Geometry: final body of the model. Coordinates: model frame, mm. Face numbers are marked on the shaded views. Give positions to 0.01 mm unless a question says otherwise; leave off trailing zeros. Order: outer loops, then holes, each group sorted by start corner. A loop starts at its lowest first (then second) coordinate and runs counter-clockwise, first axis right, second up. Notation, with made-up numbers: (-16, -37.5) - (10, -37.5) arc R19 cw to (10, -19.5) - close; hole circle Ø3 at (66.25, -30). An arc over 180 degrees is marked (long way). One line per item, written item: value.
```python
from build123d import *

# Parameters (mm, degrees)
F1_DEPTH = 3.302
F3_DEPTH = 1.524
F4_SIZE  = 2.54
F5_DEPTH = 1.27


with BuildPart() as f1:
    # F0 (on Top) → F1 (new body)
    with BuildSketch(Plane.XY):
        Polygon((9.3258451213, 12.835924618), (-9.3258451213, 12.835924618), (-15.08953438, -4.9028869271), (0, -15.866075382), (15.08953438, -4.9028869271), align=None)
    extrude(amount=F1_DEPTH)

    # F2 (on face) → F3 (cut)
    with BuildSketch(Plane.XY.offset(3.302)):
        Polygon((7.3849782182, 10.1645505026), (-7.3849782182, 10.1645505026), (-11.9491457632, -3.8825128116), (0, -12.564075382), (11.9491457632, -3.8825128116), align=None)
        Polygon((-9.3258451213, -4.0431052044), (-7.3849782182, 6.9842811825), (0, 6.9842811825), (7.3849782182, 6.9842811825), (9.3258451213, -4.0431052044), (4.6629225606, -2.0215526022), (0, -10.1645505026), (-4.6629225606, -2.0215526022), align=None, mode=Mode.SUBTRACT)
    extrude(amount=-F3_DEPTH, mode=Mode.SUBTRACT)

    # F4
    f4_edges = [f1.edges().sort_by_distance(p)[0] for p in [
        (7.544767, -10.384481, 3.302),
        (-7.544767, -10.384481, 3.302),
        (-12.20769, 3.966519, 3.302),
        (0, 12.835925, 3.302),
        (12.20769, 3.966519, 3.302),
    ]]
    chamfer(f4_edges, length=F4_SIZE)

    # F5 (cut): a face of the model
    f5_faces = [f1.faces().sort_by_distance(p)[0] for p in [
        (6.0321565972, -8.3025512818, 3.302),
    ]]
    extrude(f5_faces, amount=-F5_DEPTH, mode=Mode.SUBTRACT)


solid = f1.part
```
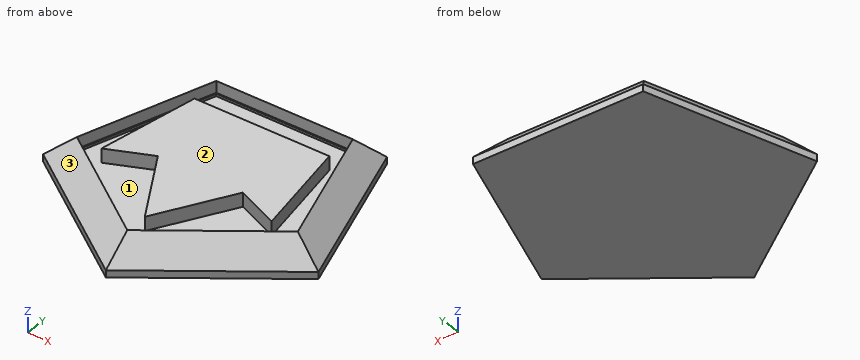
1) First-contact query: pin 1 (0.8 mm diameter, centred on x = -1, z = 2.5, fed in from +Y); pin 2 (1 mm diameter, centred on x = -9.5, y = 5, fed in from +Z). Flat tips, straight axial feed; report the tip coordinate or a pass-through.
Answers below:
pin 1: y = 11.5
pin 2: z = 3.3
2) Material intervals for line 1 along X through (y, z) = (1.75, 3); line 2 along Y through (x, z) = (5, 2.45); line 3 along X through (y, z) = (5.25, 2.65), sorted ascending.
Answers below:
line 1: -10.57 to -10.26, -8.31 to 8.31, 10.26 to 10.57
line 2: -10.15 to -9.09, -2.17 to 6.98, 10.3 to 11.15
line 3: -9.81 to -9.12, -7.69 to 7.69, 9.12 to 9.81
3) Section B-B, the plane x = -6. Return loops of the section in (y, z), then the cut area to 3 significant figures.
Answers below:
outline: (-11.51, 0) - (12.84, 0) - (12.84, 0.76) - (10.3, 3.3) - (10.3, 2.03) - (10.16, 2.03) - (10.16, 1.78) - (6.98, 1.78) - (6.98, 3.3) - (-2.6, 3.3) - (-2.6, 1.78) - (-8.2, 1.78) - (-8.2, 2.03) - (-8.37, 2.03) - (-8.37, 3.3) - (-11.51, 0.76) - close
area: 59.4 mm^2
4) Section C-C, the plane y = -11. Return loops of the section in (x, z), then the cut area to 3 significant figures.
Answers below:
outline: (-6.7, 0) - (6.7, 0) - (6.7, 0.76) - (2.38, 3.3) - (2.38, 2.03) - (2.15, 2.03) - (2.15, 1.78) - (-2.15, 1.78) - (-2.15, 2.03) - (-2.38, 2.03) - (-2.38, 3.3) - (-6.7, 0.76) - close
area: 26.1 mm^2
5) Mould query, pull axis X, two halves, no side actions, for the marked faces 1, 2 and 3. Classes: released by +X, released by -X, zero draft, split by the parting line, or undercut.
Answers below:
face 1: undercut
face 2: zero draft
face 3: released by -X
6) Section A-A, the plane z = 2.5. Return loops of the section in (x, y).
Answers below:
outline: (-13.05, -4.24) - (0, -13.72) - (13.05, -4.24) - (8.06, 11.1) - (-8.06, 11.1) - close; (-9.33, -4.04) - (-4.66, -2.02) - (0, -10.16) - (4.66, -2.02) - (9.33, -4.04) - (7.38, 6.98) - (-7.38, 6.98) - close; hole (-12.1, -3.93) - (0, -12.73) - (12.1, -3.93) - (7.48, 10.3) - (-7.48, 10.3) - close
7) Section D-D, the plane x = 12.5. Return loops of the section in (y, z).
Answers below:
outline: (-6.78, 0) - (3.07, 0) - (3.07, 0.76) - (-4.06, 2.96) - (-6.78, 0.76) - close
